Can you work these out from the model? Positions are in its coordinate system, mm. A direction names the side the tool comes from. Coordinates: 2 decimals unless noted, no trailing zeros. Loops run counter-clockwise (first coordinate to the right, second up) from the corner with the lowest first, then second, coordinate; pieces in that order, holes last. Notation, with made-up numbers: (-24, 27.25) - (5, 27.25) arc R20 cw to (5, 58.25) - close; hole circle Ø5 at (69, 50.5). An arc over 180 degrees is marked (long way). Put each result on its own line as item: value. Start each with the question number.
from build123d import *

# Parameters (mm, degrees)
F0_R     = 5
F0_W     = 40
F0_H     = 25
F0_W_2   = 20
F1_DEPTH = 10


with BuildPart() as f1:
    # F0 (on Top) → F1 (new body)
    with BuildSketch(Plane.XY):
        Polygon((-26.600002, 18.249999), (-66.600002, 18.249999), (-66.600002, -6.750001), (-46.600002, -6.750001), (-26.600002, -6.750001), align=None)
        with Locations((-46.600002, 5.749999)):
            Circle(F0_R, mode=Mode.SUBTRACT)
        with Locations((-6.600002, 5.749999)):
            Rectangle(F0_W, F0_H)
        with Locations((-6.600002, 5.749999)):
            Circle(F0_R, mode=Mode.SUBTRACT)
        with Locations((-36.600002, -19.250001)):
            Rectangle(F0_W_2, F0_H)
    extrude(amount=F1_DEPTH)


solid = f1.part
Q1. We'd pull the mould along X, two halves only. Please class faces 4 (the flat face through (-26, 18.25, 5)), 5 (the flat face through (13.4, 6, 5)), 6 (the cylindrical face through (-7.68, 0.87, 4.93)): released by +X, released by -X, zero draft, split by the parting line, or undercut.
Q2. Please list where these lines run through material, in increasing order: line 1 along X through (y, z) = (2, 6); line 2 along X through (y, z) = (5, 4.5); line 3 along Y through (x, z) = (3.5, 0.75). Write a range as [from, to].
Q3. I want a section at B-B on z = 4.75. List the corners of the cut face in (x, y) for me.
Q4. Will these pins go through, and if not, where does the flat tip stop? pin 1 (3 mm diameter, centred on y = -19.5, z = 5.5, fed in from -X); pin 2 (1 mm diameter, centred on y = -10, z = 5, fed in from +X).
Q5. I want a section at A-A on x = -4.5. List the corners of the cut face in (y, z) for me.
Q6. I want a section at C-C on y = 7.5. List the corners of the cut face in (x, z) for me, and give its area (3 significant figures).
Q7. I want a section at D-D on y = -12. List the corners of the cut face in (x, z) for me.
Q8. On a 3-axis mill with a long thin cutter (end or side, diameter ignored), from which of +Z, -Z, +X, -X, +Y, -Y can I reach the whole of each face in a straight line? I mean faces 1 (the flat face through (-7, -6.75, 5)), 2 (the flat face through (-46.6, -19, 5)), 3 (the flat face through (-27, -1, 0)). Say none if no direction works.
Calculated:
1. face 4: zero draft
1. face 5: released by +X
1. face 6: undercut
2. line 1: [-66.6, -49.91], [-43.29, -9.91], [-3.29, 13.4]
2. line 2: [-66.6, -51.54], [-41.66, -11.54], [-1.66, 13.4]
2. line 3: [-6.75, 18.25]
3. outline: (-66.6, -6.75) - (-46.6, -6.75) - (-46.6, -31.75) - (-26.6, -31.75) - (-26.6, -6.75) - (13.4, -6.75) - (13.4, 18.25) - (-66.6, 18.25) - close; hole circle Ø10 at (-46.6, 5.75); hole circle Ø10 at (-6.6, 5.75)
4. pin 1: x = -46.6
4. pin 2: x = -26.6
5. outline: (-6.75, 0) - (1.21, 0) - (1.21, 10) - (-6.75, 10) - close; (10.29, 0) - (18.25, 0) - (18.25, 10) - (10.29, 10) - close
6. outline: (-66.6, 0) - (-51.28, 0) - (-51.28, 10) - (-66.6, 10) - close; (-41.92, 0) - (-11.28, 0) - (-11.28, 10) - (-41.92, 10) - close; (-1.92, 0) - (13.4, 0) - (13.4, 10) - (-1.92, 10) - close
6. area: 613 mm2
7. outline: (-46.6, 0) - (-26.6, 0) - (-26.6, 10) - (-46.6, 10) - close
8. face 1: +Z, -Z, +X, -Y
8. face 2: +Z, -Z, -X, -Y
8. face 3: -Z, +X, -X, +Y, -Y
